Design review of the part shown in the three views and the two pictorial views. Dimensions are in mm from the part's minimum x, y and z. A direction names the side the tool comes from. Round coordinates to 2 decimals unless told otherwise and drop trailing zeros. Write each loop counter-clockwise with the first axis right and the second up, starting at its lowest first coordinate (ties: lowest second). Pieces come first, ordered by that corner, then holes. Notation, with made-up numbers: (55.25, 39.25) - (109.25, 39.25) arc R24 ccw to (109.25, 54.25) - close; hole circle Ø9 at (50, 81.25). An arc over 180 degrees is marked (long way). One line per item, written item: value. Start each with the question number.
Q1. Add section C-C on z = 3.9. Write out the cut boundary in (x, y).
Q2. Tool access review of the marked faces 1 and 2: name each direction out of +Z, -Z, +X, -X, +Y, -Y from which nothing blocks a thin tool from reaching the whole face with its end or side.
Q3. Mouldability with a two-part tool opening along Z and no side actions: class the marked faces 3, 4 and 5 as +Z half, -Z half, draft (parallel to the pull), parting line (faces both ways), or undercut.
Q4. Add section A-A on y = 1.25. Write out the cut boundary in (x, z), and give its area (3 significant figures).
Q5. Add section D-D on y = 2.6. Write out the cut boundary in (x, z), and give its area (3 significant figures).
Q6. Add section B-B on x = 3.9. Write out the cut boundary in (y, z).
Q7. For probe 1 along Z at (x, y) = (3.75, 2.05); probe 2 along Y at (x, z) = (7.25, 2); probe 3 along Y at (x, z) = (5.75, 5.5), list the stretches that pass through material, from the lowest coordinate up.
Q8. Clearance check with a flat-ended pin moving along its axis: pin 1 Ø1.4 at (x, z) = (4, 3.5) entering from -Y. State where the tip first meets the part, or that it passes through.
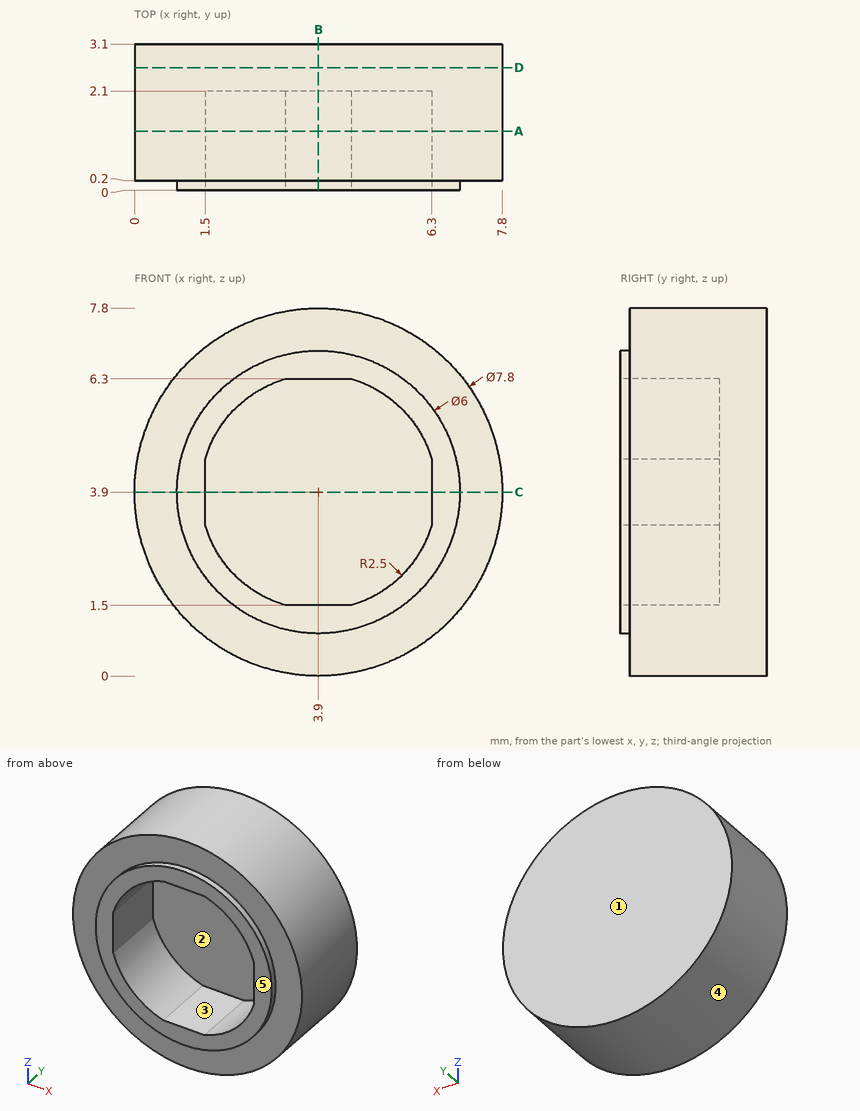
Result set:
1. outline: (0, 0.2) - (0.9, 0.2) - (0.9, 0) - (1.5, 0) - (1.5, 2.1) - (6.3, 2.1) - (6.3, 0) - (6.9, 0) - (6.9, 0.2) - (7.8, 0.2) - (7.8, 3.1) - (0, 3.1) - close
2. face 1: +Z, -Z, +X, -X, +Y
2. face 2: -Y
3. face 3: undercut
3. face 4: parting line
3. face 5: draft
4. outline: circle Ø7.8 at (3.9, 3.9); hole (1.5, 3.2) arc R2.5 ccw to (3.2, 1.5) - (4.6, 1.5) arc R2.5 ccw to (6.3, 3.2) - (6.3, 4.6) arc R2.5 ccw to (4.6, 6.3) - (3.2, 6.3) arc R2.5 ccw to (1.5, 4.6) - close
4. area: 28.5 mm^2
5. outline: circle Ø7.8 at (3.9, 3.9)
5. area: 47.8 mm^2
6. outline: (0, 0.9) - (0.2, 0.9) - (0.2, 0) - (3.1, 0) - (3.1, 7.8) - (0.2, 7.8) - (0.2, 6.9) - (0, 6.9) - (0, 6.3) - (2.1, 6.3) - (2.1, 1.5) - (0, 1.5) - close
7. probe 1: z = 0 to 1.5, 6.3 to 7.8
7. probe 2: y = 0.2 to 3.1
7. probe 3: y = 2.1 to 3.1
8. pin 1: stops at y = 2.1
